from build123d import *

# Parameters (mm, degrees)
F1_DEPTH = 10
F2_T     = -3
F3_R     = 5


with BuildPart() as f1:
    # F0 (on Top) → F1 (new body)
    with BuildSketch(Plane.XY):
        with BuildLine():
            ThreePointArc((-28, 60), (-32.949747, 57.949747), (-35, 53))
            Line((-35, 53), (-35, 0))
            Line((-35, 0), (-35, -53))
            ThreePointArc((-35, -53), (-32.949747, -57.949747), (-28, -60))
            Line((-28, -60), (28, -60))
            ThreePointArc((28, -60), (32.949747, -57.949747), (35, -53))
            Line((35, -53), (35, 0))
            Line((35, 0), (35, 53))
            ThreePointArc((35, 53), (32.949747, 57.949747), (28, 60))
            Line((28, 60), (0, 60))
            Line((0, 60), (-28, 60))
        make_face()
    extrude(amount=F1_DEPTH)

    # F2
    f2_openings = [f1.faces().sort_by_distance(p)[0] for p in [
        (0, 0, 0),
    ]]
    offset(amount=F2_T, openings=f2_openings)

    # F3
    f3_edges = [f1.edges().sort_by_distance(p)[0] for p in [
        (-32.949747, 57.949747, 10),
    ]]
    fillet(f3_edges, radius=F3_R)


solid = f1.part
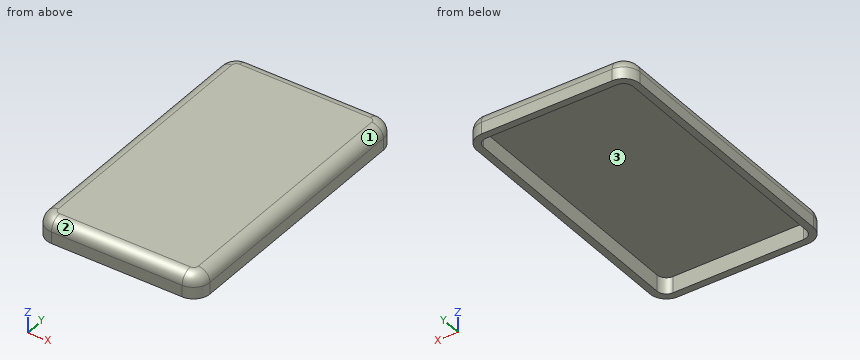
Input: part model. Units: mm. Frame: model coordinates. Face numbers are marked on the shaded views. Give positions to 0.01 mm unless a question says otherwise; leave off trailing zeros. Order: outer loops, then holes, each group sorted by start corner. A loop starts at its lowest first (then second) coordinate and runs counter-clockwise, first axis right, second up. Notation, with made-up numbers: (-5, 80.25) -> (21, 80.25) arc R24 ccw to (21, 112.25) -> close; hole circle Ø11 at (10, 58). An arc over 180 degrees is marked (long way). Use one line per item in the form item = value.
1) Line query: probe 1 along Y at (x, z) = (-26.5, 5.25); probe 2 along X at (y, z) = (-15.5, 0.75); probe 3 along Z at (x, y) = (-15.5, 15). Output: solid intervals per line, ascending.
Response values:
probe_1 = -59.99 to -57, 57 to 59.99
probe_2 = -35 to -32, 32 to 35
probe_3 = 7 to 10
2) First-contact query: pin 1 Ø1.5 at (y, z) = (-18.5, 6.5) entering from -X; pin 2 Ø1 at (x, y) = (12.5, -18.5) entering from -Z; pin 3 Ø2 at (x, z) = (5.5, 8) entering from -Y. Flat tips, straight axial feed; report the tip coordinate or a pass-through.
Response values:
pin_1 = -34.94
pin_2 = 7
pin_3 = -59.58
3) Mould query, pull axis Y, two halves, no side actions, for the marked faces 1, 2 and 3. Classes: pulls with the +Y half, pulls with the -Y half, needs draft (parallel to the pull), parting line crosses it, or undercut.
Response values:
face_1 = needs draft
face_2 = pulls with the -Y half
face_3 = undercut
4) Section A-A, the plane x = 21. Return loops of the section in (y, z).
Response values:
outline = (-60, 0) -> (-57, 0) -> (-57, 7) -> (57, 7) -> (57, 0) -> (60, 0) -> (60, 5) arc R5 ccw to (55, 10) -> (-55, 10) arc R5 ccw to (-60, 5) -> close
5) Section B-B, the plane y = -29. Return loops of the section in (x, z), and give its area (3 significant figures).
Response values:
outline = (-35, 0) -> (-32, 0) -> (-32, 7) -> (32, 7) -> (32, 0) -> (35, 0) -> (35, 5) arc R5 ccw to (30, 10) -> (-30, 10) arc R5 ccw to (-35, 5) -> close
area = 241 mm^2
